from build123d import *

# Parameters (mm, degrees)
SKETCH_1_R               = 1.5
EXTRUDE_606_DEPTH        = 8
CHAMFER_689_SIZE         = 0.5
CUT_EXTRUDE_1_DEPTH      = 0.28
PATTERN_CIRCULAR_1_COUNT = 2
PATTERN_CIRCULAR_1_ANGLE = 90


with BuildPart() as part:
    # Эскиз1 → Extrude 606 (new body)
    with BuildSketch(Plane(origin=(0, 0, 0), x_dir=(0, 0, -1), z_dir=(1, 0, 0))):
        Circle(SKETCH_1_R)
    extrude(amount=-EXTRUDE_606_DEPTH)

    # Chamfer 689
    chamfer_689_edges = [part.edges().sort_by_distance(p)[0] for p in [
        (-8, 0, 1.5),
    ]]
    chamfer(chamfer_689_edges, length=CHAMFER_689_SIZE)

    # Эскиз7 → Revolve 901 (revolve)
    with BuildSketch(Plane.XY, mode=Mode.PRIVATE) as revolve_901_sk:
        Polygon((0, 0), (0, 2.8), (-0.35, 2.8), (-1.65, 1.5), (-1.65, 0), align=None)
    revolve(revolve_901_sk.sketch.rotate(Axis((0, 0, 0), (-1, 0, 0)), 90), axis=Axis((0, 0, 0), (-1, 0, 0)))

    # Эскиз10 → Вырез-Вытянуть1 (cut, symmetric)
    with BuildSketch(Plane.XY):
        Polygon((0, 1.4), (0, -1.4), (-1.5, -0.652127588), (-1.697863748, -0.28), (-1.697863748, 0.28), (-1.5, 0.652127588), align=None)
    cut_extrude_1 = extrude(amount=CUT_EXTRUDE_1_DEPTH, both=True, mode=Mode.SUBTRACT)

    # Круговой массив1: Вырез-Вытянуть1 ×2 about axis
    pattern_circular_1_axis = Axis((0, 0, 0), (1, 0, 0))
    for i in range(1, PATTERN_CIRCULAR_1_COUNT):
        add(cut_extrude_1.rotate(pattern_circular_1_axis, i * PATTERN_CIRCULAR_1_ANGLE / (PATTERN_CIRCULAR_1_COUNT - 1)), mode=Mode.SUBTRACT)


solid = part.part
Source: CAD feature listing. Evaluate the final solid. Frame: model axes, mm. A direction names the side the tool comes from. Give positions to 0.01 mm unless a question says otherwise; leave off trailing zeros. Write each loop counter-clockwise with the first axis right and the second up, starting at its lowest first coordinate (ties: lowest second). Pieces come first, ordered by that corner, then holes. Notation, with made-up numbers: M 18.25,53.5 L 44.25,53.5 A26 ccw 44.25,88.5 Z; hole C -24.5,39 d9. An arc over 180 degrees is marked long. Return JSON: item names as keys, results as strings. Group by question number.
1) Set-up query: faces 4 (the face through (-4.53, 0.07, 1.5)), 5 (the face through (-0.6, -0.28, -0.7)), 6 (the face through (-8, 0, 0)). Return all of +Z, -Z, +X, -X, +Y, -Y with unobstructed straight access to the full face (end or side cutting, diameter ignored); none if empty.
2) Pin query (flat end, axial travel): P1, Ø1.2, axis at x = -1, y = -1, coming from the +Z side; P2, Ø0.6, axis at x = -0.5, y = 0.5, coming from the +Z side; P3, Ø1.2, axis at x = -1, z = 1, coming from the +Y side. Return the tip coordinate at first contact, or that it passes through.
3) Cut plane A-A, the plane y = 0. Output: boundary loops of the cut face in (x, z), plus the area to 3 significant figures.
4) Material intervals for line 1 along Y through (x, z) = (-4.5, 0.85); line 2 along Y through (x, z) = (-1.25, 0.55); line 3 along X through (y, z) = (-2.35, 0.75), sorted ascending. Write a range as [from, to].
5) Pull-direction query (Z, two-part tool) for faces 1 (the face through (-0.2, -0.1, 2.8)), 2 (the face through (-0.6, 0.28, -0.7)), 3 (the face through (0, 1, 1)); classes: pulls with the +Z half, pulls with the -Z half, needs draft (parallel to the pull), parting line crosses it, or undercut.
Recorded:
{
 "1": {"face 4": "-X", "face 5": "+X", "face 6": "+Z, -Z, -X, +Y, -Y"},
 "2": {"P1": "stops at z = 2.6", "P2": "stops at z = 2.79", "P3": "stops at y = 2.6"},
 "3": {"outline": "M -8,-1 L -7.5,-1.5 L -1.65,-1.5 L -0.35,-2.8 L 0,-2.8 L 0,-1.4 L -1.5,-0.65 L -1.7,-0.28 L -1.7,0.28 L -1.5,0.65 L 0,1.4 L 0,2.8 L -0.35,2.8 L -1.65,1.5 L -7.5,1.5 L -8,1 Z", "area": "23.1 mm²"},
 "4": {"line 1": "y = [-1.24, 1.24]", "line 2": "y = [-1.82, -0.28], [0.28, 1.82]", "line 3": "x = [-0.68, 0]"},
 "5": {"face 1": "parting line crosses it", "face 2": "undercut", "face 3": "needs draft"}
}
